Read the model definition and answer for the solid it produces. Units are mm, in the model's axes. A direction names the side the tool comes from. Coordinates: 2 decimals unless noted, no trailing zeros. Loops run counter-clockwise (first coordinate to the right, second up) from the corner with the lowest first, then second, coordinate; pieces in that order, holes last. Notation, with made-up numbers: (66, 66.5) - (91, 66.5) arc R21 cw to (91, 96.5) - close; hole circle Ø3 at (-4, -22). An arc over 180 degrees is marked (long way). Use one line per item in the form item = value.
Autodesk Inventor part; units mm, degrees
ref_plane "YZ Plane" through (0, 0, 0) normal (1, 0, 0) x (0, 1, 0)
ref_plane "XZ Plane" through (0, 0, 0) normal (0, 1, 0) x (-1, 0, 0)
ref_plane "XY Plane" through (0, 0, 0) normal (0, 0, 1) x (1, 0, 0)
sketch "Sketch1" plane through (0, 0, 0) normal (0, 0, 1) x (1, 0, 0)
  line L0 (0, 0) -> (7, 0)
  line L1 (7, 0) -> (7, 7)
  line L2 (7, 7) -> (0, 7)
  line L3 (0, 7) -> (0, 0)
  dimension "d0" = 7
  dimension "d1" = 7
extrude "Extrusion1" add sketch "Sketch1" along normal blind 3
sketch "Sketch2" plane through (0, 0, 3) normal (0, 0, 1) x (1, 0, 0)
  circle A0 centre (3.175, 3.175) radius 2.5
  point P0 (0, 0)
  dimension "d4" = 5
extrude "Extrusion2" add sketch "Sketch2" along normal blind 15
thread "Thread1"
properties part number "AD"
Item 1: Each of these flat-tipped pins is pushed along its axis until it touches: P1, Ø1, axis at y = 3.5, z = 5.5, coming from the +X side (3 decimals); P2, Ø1, axis at y = 5.5, z = 14, coming from the +X side; P3, Ø1, axis at x = 6.5, y = 4, coming from the +Z side. Where does it stop, or does it pass through?
Results below:
P1 = 5.675
P2 = 4.88
P3 = 3
Item 2: Which of the six approach directions +Z, -Z, +X, -X, +Y, -Y give full straight-line access (tool end or side, diameter ignored) to faces 1 (the flat face through (4, 7, 1)), 2 (the flat face through (5, 5.1, 3))?
Results below:
face_1 = +Z, -Z, +X, -X, +Y
face_2 = +Z
Item 3: Find the intervals of material crossed by L1, parallel to Z at x = 3.75, y = 6; L2, parallel to X at y = 1.5, z = 9.25; L3, parallel to Y at x = 2.5, z = 4, in increasing order.
Results below:
L1 = 0 to 3
L2 = 1.32 to 5.03
L3 = 0.77 to 5.58
Item 4: The part is cut by section B-B on y = 3.5. Give the vertices of the cut face in (x, z).
Results below:
outline = (0, 0) - (7, 0) - (7, 3) - (5.65, 3) - (5.65, 18) - (0.7, 18) - (0.7, 3) - (0, 3) - close
Item 5: The part is cut by section C-C on z = 6.75. Give the vertices of the cut face in (x, y) (3 decimals), plus the area to 3 significant figures.
Results below:
outline = circle Ø5 at (3.175, 3.175)
area = 19.6 mm²
Item 6: The part is cut by section A-A on x = 4.25. Give the vertices of the cut face in (y, z).
Results below:
outline = (0, 0) - (7, 0) - (7, 3) - (5.43, 3) - (5.43, 18) - (0.92, 18) - (0.92, 3) - (0, 3) - close
Item 7: The part is cut by section D-D on y = 6. Give the vertices of the cut face in (x, z), plus the area to 3 significant figures.
Results below:
outline = (0, 0) - (7, 0) - (7, 3) - (0, 3) - close
area = 21.0 mm²
